```python
from build123d import *

# Parameters (mm, degrees)
F1_DEPTH = 63.5
F0_W     = 25.3785441501
F0_H     = 19.05
F2_DEPTH = 25.4
F3_DEPTH = 7.9375
F5_R     = 5.08


with BuildPart() as f1:
    # F0 (on Front) → F1 (new body, symmetric)
    with BuildSketch(Plane.XZ):
        Polygon((41.275, -9.525), (41.275, 9.525), (22.225, 9.525), (-41.275, 9.525), (-41.275, -9.525), align=None)
    extrude(amount=F1_DEPTH, both=True)

    # F0 (on Front) → F2 (join, symmetric)
    with BuildSketch(Plane.XZ):
        with Locations((70.927461476, 52.4002)):
            Rectangle(F0_W, F0_H)
        with BuildLine():
            Line((22.225, 9.525), (41.275, 9.525))
            Line((41.275, 9.525), (41.275, 27.0002))
            ThreePointArc((41.275, 27.0002), (45.9246798487, 38.2255201513), (57.15, 42.8752))
            Line((57.15, 42.8752), (58.2381894009, 42.8752))
            Line((58.2381894009, 42.8752), (58.2381894009, 61.9252))
            Line((58.2381894009, 61.9252), (57.15, 61.9252))
            ThreePointArc((57.15, 61.9252), (32.4542956671, 51.6959043329), (22.225, 27.0002))
            Line((22.225, 27.0002), (22.225, 9.525))
        make_face()
    extrude(amount=F2_DEPTH, both=True)

    # F0 (on Front) → F3 (join, symmetric)
    with BuildSketch(Plane.XZ):
        with BuildLine():
            Line((-41.275, 9.525), (22.225, 9.525))
            Line((22.225, 9.525), (22.225, 27.0002))
            ThreePointArc((22.225, 27.0002), (32.4542956671, 51.6959043329), (57.15, 61.9252))
            add(Edge.make_bspline(
                [(-41.275, 9.525), (-24.9403305352, 44.9881963432), (34.9694043398, 64.3845573068), (57.15, 61.9252)],
                knots=[0, 0, 0, 0, 111.5045361635, 111.5045361635, 111.5045361635, 111.5045361635], degree=3))
        make_face()
    extrude(amount=F3_DEPTH, both=True)

    # F0 (on Front) → F4 (revolve)
    with BuildSketch(Plane.XZ):
        Polygon((83.616733551, 61.9252), (83.616733551, 42.8752), (83.616733551, 38.1), (109.0381894009, 38.1), (109.0381894009, 66.675), (83.616733551, 66.675), align=None)
    revolve(axis=Axis((83.616733551, 0, 52.3875), (0, 0, -1)))

    # F5
    f5_edges = [f1.edges().sort_by_distance(p)[0] for p in [
        (-41.275, -63.5, 0),
        (-41.275, 63.5, 0),
        (41.275, 63.5, 0),
        (41.275, -63.5, 0),
    ]]
    fillet(f5_edges, radius=F5_R)


solid = f1.part
```
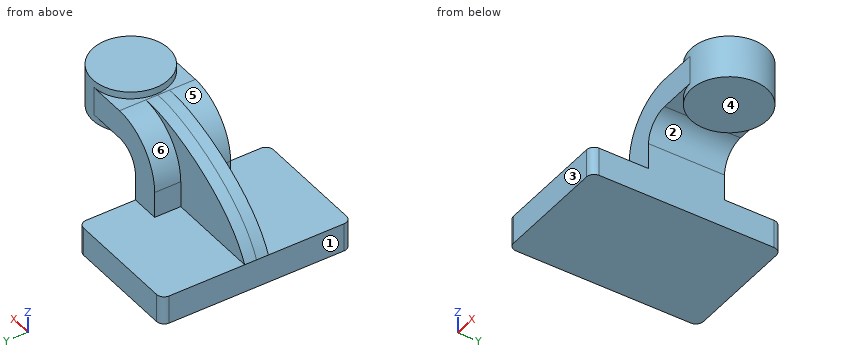
Geometry check sheet. Reference: the model listing, model coordinates, mm. Face numbers are marked on the shaded views. A direction names the side the tool comes from. Coordinates: 2 decimals unless noted, no trailing zeros. Order: outer loops, then holes, each group sorted by start corner. A loop starts at its lowest first (then second) coordinate and runs counter-clockwise, first axis right, second up. Notation, with made-up numbers: (77.25, -8) - (101.25, -8) arc R23 ccw to (101.25, 18) - close; hole circle Ø9 at (29, 4). An arc over 180 degrees is marked (long way). Answer in a Markdown table with one row per item. Add a question column.
1. Draft check along X on the marked faces 1, 2 and 3. Enter one of: +X half, -X half, draft (parallel to the pull), parting line (faces both ways), or undercut.
2. Access from +Z, -Z, +X, -X, +Y, -Y to the whole of each face (thin tool, end or side, straight path). Record for the marked faces 4, 5 and 6.
3. Section check B-B (y = -47). Enter the section's corners in (x, z) (3 decimals).
4. Section check A-A (y = 15). Enter the section's corners in (x, z) (3 decimals), plus the area to 3 significant figures.
5. Material ranges on L1, parallel to Y at x = -8, z = 27.5; L2, parallel to Z at x = 4.5, y = 28.5 (3 decimals); L3, parallel to X at y = 23, z = 10.5 (3 decimals), recorded low to high. Write a range as [from, to].
6. Gauge pin test, flat ends, axial feed: pin 1 Ø16.5 at (x, y) = (-7.5, -37.5) entering from +Z (3 decimals); pin 2 Ø14 at (y, z) = (15, 20.5) entering from -X (3 decimals); pin 3 Ø15.5 at (x, y) = (76, -2.5) entering from -Z. Record the tip position at first contact, or that the pin passes through.
Data:
| question | item | result |
|---|---|---|
| 1 | face 1 | -X half |
| 1 | face 2 | undercut |
| 1 | face 3 | draft |
| 2 | face 4 | -Z, +X, +Y, -Y |
| 2 | face 5 | +Z, -X, -Y |
| 2 | face 6 | +Z, -X, +Y |
| 3 | outline | (-41.275, -9.525) - (41.275, -9.525) - (41.275, 9.525) - (-41.275, 9.525) - close |
| 4 | outline | (-41.275, -9.525) - (41.275, -9.525) - (41.275, 27) arc R15.875 cw to (57.15, 42.875) - (63.092, 42.875) - (63.092, 38.1) - (104.141, 38.1) - (104.141, 66.675) - (63.092, 66.675) - (63.092, 61.925) - (57.15, 61.925) arc R34.925 ccw to (22.225, 27) - (22.225, 9.525) - (-41.275, 9.525) - close |
| 4 | area | 3,950 mm² |
| 5 | L1 | y = [-7.94, 7.94] |
| 5 | L2 | z = [-9.525, 9.525] |
| 5 | L3 | x = [22.225, 41.275] |
| 6 | pin 1 | stops at z = 9.525 |
| 6 | pin 2 | stops at x = 22.225 |
| 6 | pin 3 | stops at z = 38.1 |
